Part model, mm, in its own coordinate system. A direction names the side the tool comes from. Give positions to 0.01 mm unless a question says otherwise; leave off trailing zeros. Write each loop counter-clockwise with the first axis right and the second up, starting at its lowest first coordinate (ties: lowest second). Pieces come first, ordered by that corner, then holes.
Autodesk Inventor part; units mm, degrees
ref_plane "YZ Plane" through (0, 0, 0) normal (1, 0, 0) x (0, 1, 0)
ref_plane "XZ Plane" through (0, 0, 0) normal (0, 1, 0) x (-1, 0, 0)
ref_plane "XY Plane" through (0, 0, 0) normal (0, 0, 1) x (1, 0, 0)
sketch "Sketch1" plane through (0, 0, 0) normal (0, 1, 0) x (-1, 0, 0)
  line L0 (-128.5875, 95.25) -> (128.5875, 95.25)
  line L1 (128.5875, 95.25) -> (128.5875, -95.25)
  line L2 (128.5875, -95.25) -> (-128.5875, -95.25)
  line L3 (-128.5875, -95.25) -> (-128.5875, 95.25)
  line L4 (-128.5875, 95.25) -> (128.5875, -95.25) construction
  line L5 (128.5875, 95.25) -> (-128.5875, -95.25) construction
  line L6 (-115.8875, 82.55) -> (115.8875, 82.55)
  line L7 (115.8875, 82.55) -> (115.8875, -82.55)
  line L8 (115.8875, -82.55) -> (-115.8875, -82.55)
  line L9 (-115.8875, -82.55) -> (-115.8875, 82.55)
  line L10 (-115.8875, 82.55) -> (115.8875, -82.55) construction
  line L11 (115.8875, 82.55) -> (-115.8875, -82.55) construction
  line L12 (134.9375, -101.6) -> (134.9375, 101.6)
  line L13 (134.9375, 101.6) -> (-134.9375, 101.6)
  line L14 (-134.9375, 101.6) -> (-134.9375, -101.6)
  line L15 (-134.9375, -101.6) -> (134.9375, -101.6)
  point P0 (0, 0)
  point P1 (0, 0)
  dimension "d0" = 231.775
  dimension "d1" = 12.7
  dimension "d2" = 12.7
  dimension "d3" = 165.1
  dimension "d4" = 6.35
extrude "Extrusion1" add sketch "Sketch1" along normal blind 60 contours L15 L14 L13 L12
extrude "Extrusion2" add sketch "Sketch1" against normal blind 15.24 contours L0 L1 L2 L3 | L6 L7 L8 L9 | L15 L14 L13 L12
fillet "Fillet1" radius 25.4 4 edges at (128.5875, 30, 95.25) (-128.5875, 30, 95.25) (-128.5875, 30, -95.25) (128.5875, 30, -95.25)
sketch "Sketch2" plane through (0, 0, 0) normal (0, 1, 0) x (1, 0, 0)
  line L0 (28.575, -88.9) -> (-28.575, -88.9)
  line L1 (-28.575, 88.9) -> (28.575, 88.9)
  arc A0 (28.575, -88.9) -> (28.575, 88.9) centre (28.575, 0) ccw
  arc A1 (-28.575, 88.9) -> (-28.575, -88.9) centre (-28.575, 0) ccw
  line L2 (28.575, 76.2) -> (-28.575, 76.2)
  arc A2 (-28.575, 76.2) -> (-28.575, -76.2) centre (-28.575, 0) ccw
  line L3 (-28.575, -76.2) -> (28.575, -76.2)
  arc A3 (28.575, -76.2) -> (28.575, 76.2) centre (28.575, 0) ccw
  line L4 (-28.575, 63.5) -> (28.575, 63.5)
  arc A4 (28.575, -63.5) -> (28.575, 63.5) centre (28.575, 0) ccw
  line L5 (28.575, -63.5) -> (-28.575, -63.5)
  arc A5 (-28.575, 63.5) -> (-28.575, -63.5) centre (-28.575, 0) ccw
  line L6 (28.575, 50.8) -> (-28.575, 50.8)
  arc A6 (-28.575, 50.8) -> (-28.575, -50.8) centre (-28.575, 0) ccw
  line L7 (-28.575, -50.8) -> (28.575, -50.8)
  arc A7 (28.575, -50.8) -> (28.575, 50.8) centre (28.575, 0) ccw
  line L8 (-28.575, 38.1) -> (28.575, 38.1)
  arc A8 (28.575, -38.1) -> (28.575, 38.1) centre (28.575, 0) ccw
  line L9 (28.575, -38.1) -> (-28.575, -38.1)
  arc A9 (-28.575, 38.1) -> (-28.575, -38.1) centre (-28.575, 0) ccw
  line L10 (28.575, 25.4) -> (-28.575, 25.4)
  arc A10 (-28.575, 25.4) -> (-28.575, -25.4) centre (-28.575, 0) ccw
  line L11 (-28.575, -25.4) -> (28.575, -25.4)
  arc A11 (28.575, -25.4) -> (28.575, 25.4) centre (28.575, 0) ccw
  line L12 (-28.575, 12.7) -> (28.575, 12.7)
  arc A12 (28.575, -12.7) -> (28.575, 12.7) centre (28.575, 0) ccw
  line L13 (28.575, -12.7) -> (-28.575, -12.7)
  arc A13 (-28.575, 12.7) -> (-28.575, -12.7) centre (-28.575, 0) ccw
  circle A14 centre (0, 0) radius 5.715
  point P0 (0, 12.7)
  dimension "d10" = 88.9
  dimension "d11" = 57.15
  dimension "d12" = 12.7
  dimension "d13" = 12.7
  dimension "d14" = 12.7
  dimension "d15" = 12.7
  dimension "d17" = 12.7
  dimension "d18" = 12.7
  dimension "d19" = 11.43
extrude "Extrusion3" cut sketch "Sketch2" against normal through all contours A14
extrude "Extrusion4" cut sketch "Sketch2" against normal blind 3.175
sketch "Sketch3" plane through (0, 0, 0) normal (0, 1, 0) x (1, 0, 0)
  arc A0 (128.5875, 69.85) -> (103.1875, 95.25) centre (103.1875, 69.85) ccw
  line L0 (103.1875, 95.25) -> (-103.1875, 95.25)
  arc A1 (-103.1875, 95.25) -> (-128.5875, 69.85) centre (-103.1875, 69.85) ccw
  line L1 (-128.5875, 69.85) -> (-128.5875, -69.85)
  arc A2 (-128.5875, -69.85) -> (-103.1875, -95.25) centre (-103.1875, -69.85) ccw
  line L2 (-103.1875, -95.25) -> (103.1875, -95.25)
  arc A3 (103.1875, -95.25) -> (128.5875, -69.85) centre (103.1875, -69.85) ccw
  line L3 (128.5875, -69.85) -> (128.5875, 69.85)
  arc A4 (28.575, -88.9) -> (28.575, 88.9) centre (28.575, 0) ccw
  line L4 (28.575, -88.9) -> (-28.575, -88.9)
  arc A5 (-28.575, 88.9) -> (-28.575, -88.9) centre (-28.575, 0) ccw
  line L5 (-28.575, 88.9) -> (28.575, 88.9)
  line L6 (-12.7, -88.9) -> (12.7, -88.9)
  line L7 (12.7, -88.9) -> (12.7, 88.9)
  line L8 (12.7, 88.9) -> (-12.7, 88.9)
  line L9 (-12.7, 88.9) -> (-12.7, -88.9)
  line L10 (-12.7, -88.9) -> (12.7, 88.9) construction
  line L11 (12.7, -88.9) -> (-12.7, 88.9) construction
  line L12 (-28.575, 88.9) -> (28.575, 88.9)
  line L13 (103.1875, -69.85) -> (-103.1875, 69.85) construction
  circle A6 centre (0, 0) radius 5.715
  line L14 (110.3067, -59.333) -> (-96.0683, 80.367)
  line L15 (-110.3067, 59.333) -> (96.0683, -80.367)
  arc A7 (96.0683, -80.367) -> (110.3067, -59.333) centre (103.1875, -69.85) ccw
  arc A8 (-96.0683, 80.367) -> (-110.3067, 59.333) centre (-103.1875, 69.85) ccw
  line L16 (-103.1875, -69.85) -> (103.1875, 69.85) construction
  line L17 (-96.0683, -80.367) -> (110.3067, 59.333)
  line L18 (96.0683, 80.367) -> (-110.3067, -59.333)
  arc A9 (-110.3067, -59.333) -> (-96.0683, -80.367) centre (-103.1875, -69.85) ccw
  arc A10 (110.3067, 59.333) -> (96.0683, 80.367) centre (103.1875, 69.85) ccw
  dimension "d24" = 25.4
  dimension "d25" = 25.4
  dimension "d26" = 25.4
extrude "Extrusion5" cut sketch "Sketch3" against normal blind 3.175 contours L15 L7 L17 L14 A4 | A4 L14 A7 L15 | L4 L9 L17 L15 L7 | L15 L17 L7 | L17 L14 L7 L18 A4 | A4 L18 A10 L17 | L17 L7 L14 | L17 L15 L9 L18 L14 L7 | L17 L9 L15 | L17 A5 L18 L15 L9 | L14 L18 L7 | L15 L18 L9 | L17 A9 L18 A5 | L18 L14 L9 L5 L7 | L18 L9 L14 | L18 L15 A5 L14 L9 | L15 A8 L14 A5 | A6
sketch "Sketch4" plane through (0, 0, 0) normal (0, 1, 0) x (1, 0, 0)
  line L0 (-12.7, 23.9331) -> (-12.7, 25.4)
  line L1 (-12.7, 25.4) -> (-14.8671, 25.4)
  line L2 (-14.8671, 25.4) -> (-12.7, 23.9331)
  line L3 (12.7, 23.9331) -> (14.8671, 25.4)
  line L4 (14.8671, 25.4) -> (12.7, 25.4)
  line L5 (12.7, 25.4) -> (12.7, 23.9331)
  line L6 (12.7, -23.9331) -> (12.7, -25.4)
  line L7 (12.7, -25.4) -> (14.8671, -25.4)
  line L8 (14.8671, -25.4) -> (12.7, -23.9331)
  line L9 (-12.7, -25.4) -> (-12.7, -23.9331)
  line L10 (-12.7, -23.9331) -> (-14.8671, -25.4)
  line L11 (-14.8671, -25.4) -> (-12.7, -25.4)
  point P0 (0, 0)
extrude "Extrusion6" cut sketch "Sketch4" against normal blind 3.175
sketch "Sketch5" plane through (0, 60, 0) normal (0, 1, 0) x (1, 0, 0)
  line L0 (-128.5875, -69.85) -> (-128.5875, 69.85)
  arc A0 (-103.1875, 95.25) -> (-128.5875, 69.85) centre (-103.1875, 69.85) ccw
  line L1 (-103.1875, 95.25) -> (103.1875, 95.25)
  arc A1 (128.5875, 69.85) -> (103.1875, 95.25) centre (103.1875, 69.85) ccw
  line L2 (128.5875, 69.85) -> (128.5875, -69.85)
  arc A2 (103.1875, -95.25) -> (128.5875, -69.85) centre (103.1875, -69.85) ccw
  line L3 (103.1875, -95.25) -> (-103.1875, -95.25)
  arc A3 (-128.5875, -69.85) -> (-103.1875, -95.25) centre (-103.1875, -69.85) ccw
  line L4 (-134.9375, 101.6) -> (-134.9375, -101.6)
  line L5 (-134.9375, -101.6) -> (134.9375, -101.6)
  line L6 (134.9375, -101.6) -> (134.9375, 101.6)
  line L7 (134.9375, 101.6) -> (-134.9375, 101.6)
  circle A4 centre (-127.3175, 93.98) radius 3.175
  circle A5 centre (127.3175, 93.98) radius 3.175
  circle A6 centre (127.3175, -93.98) radius 3.175
  circle A7 centre (-127.3175, -93.98) radius 3.175
  point P0 (0, 0)
  dimension "d31" = 6.35
  dimension "d32" = 7.62
  dimension "d33" = 7.62
  dimension "d34" = 7.62
  dimension "d35" = 7.62
extrude "Extrusion7" cut sketch "Sketch5" against normal through all contours L0 A0 L1 A1 L2 A2 L3 A3 | L7 L6 L5 L4 | A4 | A5 | A6 | A7
extrude "Extrusion8" add sketch "Sketch5" along normal blind 6.35 contours L0 A0 L1 A1 L2 A2 L3 A3 | L7 L6 L5 L4
extrude "Extrusion9" add sketch "Sketch5" against normal blind 6.35 contours L0 A0 L1 A1 L2 A2 L3 A3
sketch "Sketch6" plane through (0, 66.35, 0) normal (0, 1, 0) x (1, 0, 0)
  circle A0 centre (-63.5, 0) radius 5.715
  circle A1 centre (63.5, 0) radius 5.715
  point P0 (0, 0)
  dimension "d42" = 63.5
  dimension "d43" = 63.5
  dimension "d44" = 11.43
  dimension "d45" = 11.43
extrude "Extrusion10" cut sketch "Sketch6" against normal through all
chamfer "Chamfer2" distance 1.5875 angle 45 8 edges at (0, 53.65, -95.25) (121.148, 53.65, -87.8105) (128.5875, 53.65, 0) (121.148, 53.65, 87.8105) (0, 53.65, 95.25) (-121.148, 53.65, 87.8105) (-128.5875, 53.65, 0) (-121.148, 53.65, -87.8105)
sketch "Sketch7" plane through (0, 53.65, 0) normal (0, -1, 0) x (1, 0, 0)
  circle A0 centre (63.5, 0) radius 5.715
  circle A1 centre (-63.5, 0) radius 5.715
  line L0 (103.1875, -93.6625) -> (-103.1875, -93.6625)
  arc A2 (103.1875, -93.6625) -> (127, -69.85) centre (103.1875, -69.85) ccw
  line L1 (127, 69.85) -> (127, -69.85)
  arc A3 (127, 69.85) -> (103.1875, 93.6625) centre (103.1875, 69.85) ccw
  line L2 (-103.1875, 93.6625) -> (103.1875, 93.6625)
  arc A4 (-103.1875, 93.6625) -> (-127, 69.85) centre (-103.1875, 69.85) ccw
  line L3 (-127, -69.85) -> (-127, 69.85)
  arc A5 (-127, -69.85) -> (-103.1875, -93.6625) centre (-103.1875, -69.85) ccw
  line L4 (-103.1875, -84.1375) -> (103.1875, -84.1375)
  arc A6 (103.1875, -84.1375) -> (117.475, -69.85) centre (103.1875, -69.85) ccw
  line L5 (117.475, -69.85) -> (117.475, 69.85)
  arc A7 (117.475, 69.85) -> (103.1875, 84.1375) centre (103.1875, 69.85) ccw
  line L6 (103.1875, 84.1375) -> (-103.1875, 84.1375)
  arc A8 (-103.1875, 84.1375) -> (-117.475, 69.85) centre (-103.1875, 69.85) ccw
  line L7 (-117.475, 69.85) -> (-117.475, -69.85)
  arc A9 (-117.475, -69.85) -> (-103.1875, -84.1375) centre (-103.1875, -69.85) ccw
  point P0 (0, 0)
  dimension "d54" = 9.525
extrude "Extrusion11" add sketch "Sketch7" along normal blind 55.3466 contours L0 A5 L3 A4 L2 A3 L1 A2
equation "\"d2\" = d1"
equation "\"d13\" = d12"
equation "\"d14\" = d13"
equation "\"d15\" = d14"
equation "\"d17\" = d15"
equation "\"d18\" = d12"
equation "\"d25\" = d24"
equation "\"d26\" = d25"
equation "\"d33\" = d32"
equation "\"d45\" = d44"
properties part number "CorollaAirFilterCaseCover"
1) Saw through at B-B (z = 0). State how many separate pieces and enclosed holes the cut face has, and give its area (3 significant figures).
Check result:
separate pieces: 3
enclosed holes: 0
area: 4,110 mm2
2) Flat gauge pins, fed straight in: P1, Ø16.5, axis at x = -14.5, y = 30.5, coming from the -Z side; P2, Ø1.4, axis at y = 57, z = -28, coming from the +X side; P3, Ø4, axis at y = 28.5, z = 30.5, coming from the -X side; P4, Ø5.5, axis at x = 127.32, z = 93.98, coming from the +Y side. Where does each tip first touch, or does it go through?
Check result:
P1: stops at z = -93.66
P2: stops at x = 128.59
P3: stops at x = -127
P4: passes through
3) Drill centre lines: L1, parallel to X at y = 64, z = -93.98; L2, parallel to X at y = 58, z = 0 (1 decimal); L3, parallel to Z at x = 76.5, y = 8. Where is each one in solid material? Low to high.
Check result:
L1: x = -134.94 to -130.49, -124.14 to 124.14, 130.49 to 134.94
L2: x = -128.6 to -69.2, -57.8 to 57.8, 69.2 to 128.6
L3: z = -93.66 to -84.14, 84.14 to 93.66
4) 3-axis set-ups, long thin cutter, end or side, ignore diameter. For faces 4 (the flat face through (127, 26, 1)), 5 (the flat face through (-127, 26, -1)), 6 (the flat face through (-117.475, 26, 1)), 7 (the cylindrical face through (-119.84, 26.36, -86.87)): which of +Z, -Z, +X, -X, +Y, -Y reach the whole face in a straight line?
Check result:
face 4: +Z, -Z, +X, -Y
face 5: +Z, -Z, -X, -Y
face 6: -Y
face 7: -Z, -X, -Y
5) Mould opens along X. For faces 1 (the flat face through (-1, 60, -98)), 2 (the cylindrical face through (-113.18, 26.36, -80.06)), 3 (the cylindrical face through (120.949, 57.652, 88.007)) say: +X half, -X half, draft (parallel to the pull), parting line (faces both ways), or undercut.
Check result:
face 1: draft
face 2: undercut
face 3: +X half
6) Saw through at D-D (x = -4.5). Write the cut outline in (y, z).
Check result:
outline: (-1.7, -93.66) - (53.65, -93.66) - (55.24, -95.25) - (60, -95.25) - (60, -101.6) - (66.35, -101.6) - (66.35, 101.6) - (60, 101.6) - (60, 95.25) - (55.24, 95.25) - (53.65, 93.66) - (-1.7, 93.66) - (-1.7, 84.14) - (53.65, 84.14) - (53.65, -84.14) - (-1.7, -84.14) - close
